Part print with two shaded views. Sizes in mm from the minimum x, y, z corner. A direction names the side the tool comes from. Give positions to 0.01 mm unless a question says otherwise; leave off trailing zeros. Write each loop counter-clockwise with the first axis right and the second up, starting at its lowest first coordinate (ties: lowest second). Pieces come first, ordered by that corner, then holes. Notation, with made-up numbers: (38, -17) -> (80, -17) arc R19 cw to (80, -9) -> close; hole circle Ø10 at (72.5, 84.25). An arc over 180 degrees is marked (long way). Use one line per item in the form item = value. Start each with the question number.
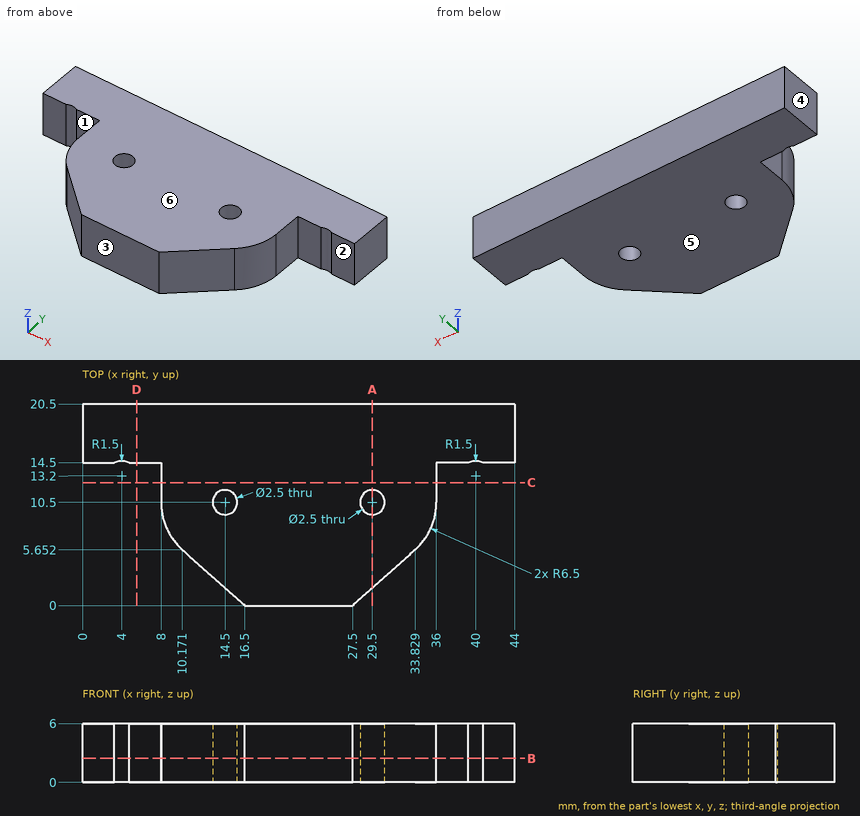
1) Pin check, flat tips, straight feed: pin 1 (1 mm diameter, centred on x = 38, z = 4, fed in from -Y); pin 2 (2 mm diameter, centred on y = 12.5, z = 2.5, fed in from -X); pin 3 (2 mm diameter, centred on x = 14.5, y = 10.5, fed in from -Z); pin 4 (1.2 mm diameter, centred on y = 13, z = 4, fed in from +X). Stop position of each tip, or through.
2) Cut at C-C (y = 12.5). Give the cut face in (x, z), and give its area (3 significant figures).
3) Wall check: line 1 along Y through (x, z) = (38.5, 5.1); line 2 along X through (y, z) = (13.75, 2.8); line 3 along Y through (x, z) = (40.5, 3.5) (1 decimal). Give the ranges that are in metal, low to high. Write a range as from..to.
4) Cut at A-A (x = 29.5). Give the cut face in (y, z).
5) Cut at B-B (z = 2.45). Give the cut face in (x, y), and give its area (3 significant figures).
6) Cut at D-D (x = 5.5). Give the cut face in (y, z), and give its area (3 significant figures).
7) 3-axis set-ups, long thin cutter, end or side, ignore diameter. For the marked faces 1, 2 and 3: which of +Z, -Z, +X, -X, +Y, -Y reach the whole face in a straight line?
8) Two-plate mould, pull along Z, no slides. Class the marked faces 4, 5 and 6: released by +Z, released by -Z, zero draft, split by the parting line, or undercut.
Final values:
q1.pin_1 = 14.5
q1.pin_2 = 8
q1.pin_3 = through
q1.pin_4 = 36
q2.outline = (8, 0) -> (36, 0) -> (36, 6) -> (8, 6) -> close
q2.area = 168 mm^2
q3.line_1 = 14.5..20.5
q3.line_2 = 8..36
q3.line_3 = 14.6..20.5
q4.outline = (1.79, 0) -> (9.25, 0) -> (9.25, 6) -> (1.79, 6) -> close; (11.75, 0) -> (20.5, 0) -> (20.5, 6) -> (11.75, 6) -> close
q5.outline = (0, 14.5) -> (3.25, 14.5) arc R1.5 cw to (4.75, 14.5) -> (8, 14.5) -> (8, 10.5) arc R6.5 ccw to (10.17, 5.65) -> (16.5, 0) -> (27.5, 0) -> (33.83, 5.65) arc R6.5 ccw to (36, 10.5) -> (36, 14.5) -> (39.25, 14.5) arc R1.5 cw to (40.75, 14.5) -> (44, 14.5) -> (44, 20.5) -> (0, 20.5) -> close; hole circle Ø2.5 at (14.5, 10.5); hole circle Ø2.5 at (29.5, 10.5)
q5.area = 593 mm^2
q6.outline = (14.5, 0) -> (20.5, 0) -> (20.5, 6) -> (14.5, 6) -> close
q6.area = 36.0 mm^2
q7.face_1 = +Z, -Z, -X, -Y
q7.face_2 = +Z, -Z, +X, -Y
q7.face_3 = +Z, -Z, +X, -X, -Y
q8.face_4 = zero draft
q8.face_5 = released by -Z
q8.face_6 = released by +Z
